Autodesk Inventor part; units mm, degrees
ref_plane "YZ Plane" through (0, 0, 0) normal (1, 0, 0) x (0, 1, 0)
ref_plane "XZ Plane" through (0, 0, 0) normal (0, 1, 0) x (-1, 0, 0)
ref_plane "XY Plane" through (0, 0, 0) normal (0, 0, 1) x (1, 0, 0)
sketch "スケッチ1" plane through (0, 0, 0) normal (0, 0, 1) x (1, 0, 0)
  arc A0 (144.025, 105.9095) -> (145.475, 108.4209) centre (142.575, 108.4209) ccw
  arc A1 (145.475, 101.5793) -> (144.025, 104.0908) centre (142.575, 101.5793) ccw
  line L0 (146, 100.67) -> (143.5, 105.0001) construction
  arc A2 (144.025, 105.9095) -> (144.025, 104.0908) centre (144.55, 105.0001) ccw
  line L1 (143.5, 105.0001) -> (146, 109.3303) construction
  circle A3 centre (148.5, 105.0001) radius 5 construction
  arc A4 (149.95, 100.67) -> (147.05, 100.67) centre (148.5, 98.1585) ccw
  line L2 (151, 100.67) -> (146, 100.67) construction
  arc A5 (145.475, 101.5793) -> (147.05, 100.67) centre (146.525, 101.5793) ccw
  arc A6 (149.95, 100.67) -> (151.525, 101.5793) centre (150.475, 101.5793) ccw
  arc A7 (152.975, 104.0908) -> (151.525, 101.5793) centre (154.425, 101.5793) ccw
  line L3 (153.5, 105.0001) -> (151, 100.67) construction
  arc A8 (152.975, 104.0908) -> (152.975, 105.9095) centre (152.45, 105.0001) ccw
  circle A9 centre (148.5, 105.0001) radius 2
  line L4 (151, 109.3303) -> (153.5, 105.0001) construction
  arc A10 (151.525, 108.4209) -> (152.975, 105.9095) centre (154.425, 108.4209) ccw
  arc A11 (151.525, 108.4209) -> (149.95, 109.3303) centre (150.475, 108.4209) ccw
  line L5 (146, 109.3303) -> (151, 109.3303) construction
  arc A12 (147.05, 109.3303) -> (149.95, 109.3303) centre (148.5, 111.8417) ccw
  arc A13 (147.05, 109.3303) -> (145.475, 108.4209) centre (146.525, 108.4209) ccw
  circle A14 centre (148.5, 105.0001) radius 6 construction
  point P0 (0, 0)
  point P1 (146, 100.67)
  point P2 (151, 100.67)
  point P3 (153.5, 105.0001)
  point P4 (145.475, 101.5793)
  point P5 (151.525, 101.5793)
  point P6 (152.975, 104.0908)
  point P7 (152.975, 105.9095)
  point P8 (151.525, 108.4209)
  point P9 (145.475, 108.4209)
  point P10 (144.025, 105.9095)
  point P11 (144.025, 104.0908)
  dimension "d4" = 10
  dimension "d5" = 360
  dimension "d6" = 360
  dimension "d7" = 1.05
  dimension "d8" = 4
  dimension "d9" = 12
extrude "押し出し1" add sketch "スケッチ1" along normal blind 5
properties part number "3ギア接続部" material "アルミニウム 2014-T4"
Check sheet for the modelled part. Datum: model origin and axes. Units: mm. Coordinates: 2 decimals unless noted, no trailing zeros. Order: outer loops, then holes, each group sorted by start corner. A loop starts at its lowest first (then second) coordinate and runs counter-clockwise, first axis right, second up. Notation, with made-up numbers: (32.5, 34.5) -> (50.5, 34.5) arc R23 ccw to (50.5, 61.5) -> close; hole circle Ø3 at (86, 47.25). An arc over 180 degrees is marked (long way). Write item = value, one per line. Start each with the question number.
1) Go/stop test with a flat-tipped pin: P1, Ø1.5, axis at x = 152, z = 1, coming from the +Y side. Record where the tip stops, or that it passes through.
2) Cross-section at D-D (x = 145). Enter the section's corners in (y, z), then the cut area to 3 significant figures.
3) Cross-section at B-B (y = 106.5). Enter the section's corners in (x, z).
4) Material ranges on L1, parallel to Y at x = 148.5, z = 2.6; L2, parallel to Y at x = 147.25, z = 2.85 (3 decimals); L3, parallel to X at y = 106, z = 0.8, recorded low to high.
5) Cross-section at A-A (x = 148.5). Enter the section's corners in (y, z).
6) Mould release check, pull along X, two halves, no side actions. Record for faces 1 (the flat face through (151, 105, 5)), 2 (the cylindrical face through (145.987, 109.322, 2.465)), 3 (the cylindrical face through (148.52, 108.94, 2.46)), 4 (the cylindrical face through (145.097, 106.989, 2.465)): +X half, -X half, draft (parallel to the pull), parting line (faces both ways), or undercut.
Ans:
q1.P1 = 109.13
q2.outline = (103.17, 0) -> (106.83, 0) -> (106.83, 5) -> (103.17, 5) -> close
q2.area = 18.3 mm²
q3.outline = (144.75, 0) -> (147.18, 0) -> (147.18, 5) -> (144.75, 5) -> close; (149.82, 0) -> (152.25, 0) -> (152.25, 5) -> (149.82, 5) -> close
q4.L1 = 101.06 to 103, 107 to 108.94
q4.L2 = 100.775 to 103.439, 106.561 to 109.225
q4.L3 = 144.17 to 146.77, 150.23 to 152.83
q5.outline = (101.06, 0) -> (103, 0) -> (103, 5) -> (101.06, 5) -> close; (107, 0) -> (108.94, 0) -> (108.94, 5) -> (107, 5) -> close
q6.face_1 = draft
q6.face_2 = undercut
q6.face_3 = undercut
q6.face_4 = -X half
